```python
from build123d import *

# Parameters (mm, degrees)
SKETCH3_W                       = 80
SKETCH3_H                       = 80
SKETCH3_W_2                     = 60
SKETCH3_H_2                     = 60
BOSS_EXTRUDE2_DEPTH             = 1550
SKETCH7_W                       = 60
SKETCH7_H                       = 60
BOSS_EXTRUDE3_DEPTH             = 5
BOSS_EXTRUDE4_REACH             = 1560.629
SKETCH8_W                       = 110
SKETCH8_H                       = 5
BOSS_EXTRUDE4_DIRECTION_2_REACH = 1560.629
CUT_EXTRUDE1_DEPTH              = 5
CUT_EXTRUDE2_REACH              = 1562.929
FILLET1_R                       = 5
FILLET1_OF_MIRROR1_R            = 5
FILLET1_OF_MIRROR2_R            = 5


with BuildPart() as part:
    # Sketch3 → Boss-Extrude2 (new body)
    with BuildSketch(Plane(origin=(0, 0, 0), x_dir=(0, 0, -1), z_dir=(1, 0, 0))):
        with Locations((40, 40)):
            Rectangle(SKETCH3_W, SKETCH3_H)
        with Locations((40, 40)):
            Rectangle(SKETCH3_W_2, SKETCH3_H_2, mode=Mode.SUBTRACT)
    extrude(amount=BOSS_EXTRUDE2_DEPTH)

    # Sketch7 → Boss-Extrude3 (add)
    with BuildSketch(Plane(origin=(1450, 0, 0), x_dir=(0, 0, -1), z_dir=(1, 0, 0))):
        Polygon((-60, 85), (140, 85), (140, 5), (90, -35), (-10, -35), (-60, 5), align=None)
        with Locations((40, 40)):
            Rectangle(SKETCH7_W, SKETCH7_H, mode=Mode.SUBTRACT)
    boss_extrude3 = extrude(amount=BOSS_EXTRUDE3_DEPTH)

    # Boss-Extrude4: up to this face of the body (flat: up to its plane)
    boss_extrude4_end = Plane(part.part.faces().sort_by_distance((1452.5, 45, -140))[0])
    # Sketch8 → Boss-Extrude4 (add, up to the picked face)
    with BuildSketch(Plane(origin=(0, 0, -80), x_dir=(-1, 0, 0), z_dir=(0, 0, -1)), mode=Mode.PRIVATE) as boss_extrude4_sk1:
        with Locations((-1400, 82.5)):
            Rectangle(SKETCH8_W, SKETCH8_H)
    boss_extrude4_tool1 = split(extrude(boss_extrude4_sk1.sketch, amount=BOSS_EXTRUDE4_REACH, mode=Mode.PRIVATE), bisect_by=boss_extrude4_end, keep=Keep.BOTH, mode=Mode.PRIVATE)
    boss_extrude4 = boss_extrude4_tool1.solids().sort_by(Axis((1400, 82.5, -80), (0, 0, -1)))[0]
    add(boss_extrude4)

    # Boss-Extrude4 direction 2: up to this face of the body (flat: up to its plane)
    boss_extrude4_direction_2_end = Plane(part.part.faces().sort_by_distance((1452.5, 45, 60))[0])
    # Sketch8 → Boss-Extrude4 direction 2 (add, up to the picked face)
    with BuildSketch(Plane(origin=(0, 0, -80), x_dir=(-1, 0, 0), z_dir=(0, 0, -1)), mode=Mode.PRIVATE) as boss_extrude4_direction_2_sk1:
        with Locations((-1400, 82.5)):
            Rectangle(SKETCH8_W, SKETCH8_H)
    boss_extrude4_direction_2_tool1 = split(extrude(boss_extrude4_direction_2_sk1.sketch, amount=-BOSS_EXTRUDE4_DIRECTION_2_REACH, mode=Mode.PRIVATE), bisect_by=boss_extrude4_direction_2_end, keep=Keep.BOTH, mode=Mode.PRIVATE)
    boss_extrude4_direction_2 = boss_extrude4_direction_2_tool1.solids().sort_by(Axis((1400, 82.5, -80), (0, 0, 1)))[0]
    add(boss_extrude4_direction_2)

    # Sketch9 → Cut-Extrude1 (cut)
    with BuildSketch(Plane(origin=(0, 85, 0), x_dir=(1, 0, 0), z_dir=(0, 1, 0))):
        with BuildLine():
            Line((1345, 80), (1350.801257358, 71.298113962))
            ThreePointArc((1350.801257358, 71.298113962), (1353.927300662, 64.675212774), (1355, 57.430609057))
            Line((1355, 57.430609057), (1355, 22.569390943))
            ThreePointArc((1355, 22.569390943), (1353.927300662, 15.324787226), (1350.801257358, 8.701886038))
            Line((1350.801257358, 8.701886038), (1345, 0))
            Line((1345, 0), (1345, 80))
        make_face()
    cut_extrude1 = extrude(amount=-CUT_EXTRUDE1_DEPTH, mode=Mode.SUBTRACT)

    # Sketch10 → Cut-Extrude2 (cut, up to next)
    with BuildSketch(Plane(origin=(0, 85, 0), x_dir=(1, 0, 0), z_dir=(0, 1, 0)), mode=Mode.PRIVATE) as cut_extrude2_sk1:
        with BuildLine():
            Line((1375, 126.5), (1425, 126.5))
            ThreePointArc((1425, 126.5), (1431.5, 120), (1425, 113.5))
            Line((1425, 113.5), (1375, 113.5))
            ThreePointArc((1375, 113.5), (1368.5, 120), (1375, 126.5))
        make_face()
    cut_extrude2_tool1 = extrude(cut_extrude2_sk1.sketch, amount=-CUT_EXTRUDE2_REACH, mode=Mode.PRIVATE) & part.part
    # Sketch10 → Cut-Extrude2 (cut, up to next)
    with BuildSketch(Plane(origin=(0, 85, 0), x_dir=(1, 0, 0), z_dir=(0, 1, 0)), mode=Mode.PRIVATE) as cut_extrude2_sk2:
        with BuildLine():
            Line((1375, -33.5), (1425, -33.5))
            ThreePointArc((1425, -33.5), (1431.5, -40), (1425, -46.5))
            Line((1425, -46.5), (1375, -46.5))
            ThreePointArc((1375, -46.5), (1368.5, -40), (1375, -33.5))
        make_face()
    cut_extrude2_tool2 = extrude(cut_extrude2_sk2.sketch, amount=-CUT_EXTRUDE2_REACH, mode=Mode.PRIVATE) & part.part
    cut_extrude2_1 = cut_extrude2_tool1.solids().sort_by_distance((1400, 85, -120))[0]
    add(cut_extrude2_1, mode=Mode.SUBTRACT)
    cut_extrude2_2 = cut_extrude2_tool2.solids().sort_by_distance((1400, 85, 40))[0]
    add(cut_extrude2_2, mode=Mode.SUBTRACT)
    cut_extrude2 = cut_extrude2_1 + cut_extrude2_2  # Cut-Extrude2 as one shape, for the pattern or mirror that repeats it

    # Fillet1
    fillet1_edges = [part.edges().sort_by_distance(p)[0] for p in [
        (1455, 85, -40),
    ]]
    fillet(fillet1_edges, radius=FILLET1_R - 0.0001)  # a hair under: the kernel refuses the full size

    # Mirror1: Boss-Extrude3 across plane
    add(boss_extrude3.mirror(Plane(origin=(775, 0, 0), x_dir=(0, 0, 1), z_dir=(1, 0, 0))))

    # Fillet1 of Mirror1
    fillet1_of_mirror1_edges = [part.edges().sort_by_distance(p)[0] for p in [
        (95, 85, -40),
    ]]
    fillet(fillet1_of_mirror1_edges, radius=FILLET1_OF_MIRROR1_R - 0.0001)  # a hair under: the kernel refuses the full size

    # Mirror2: Boss-Extrude3, Boss-Extrude4, Boss-Extrude4 direction 2, Cut-Extrude1, Cut-Extrude2 across plane
    add(boss_extrude3.mirror(Plane(origin=(775, 0, 0), x_dir=(0, 0, 1), z_dir=(1, 0, 0))))
    add(boss_extrude4.mirror(Plane(origin=(775, 0, 0), x_dir=(0, 0, 1), z_dir=(1, 0, 0))))
    add(boss_extrude4_direction_2.mirror(Plane(origin=(775, 0, 0), x_dir=(0, 0, 1), z_dir=(1, 0, 0))))
    add(cut_extrude1.mirror(Plane(origin=(775, 0, 0), x_dir=(0, 0, 1), z_dir=(1, 0, 0))), mode=Mode.SUBTRACT)
    add(cut_extrude2.mirror(Plane(origin=(775, 0, 0), x_dir=(0, 0, 1), z_dir=(1, 0, 0))), mode=Mode.SUBTRACT)

    # Fillet1 of Mirror2
    fillet1_of_mirror2_edges = [part.edges().sort_by_distance(p)[0] for p in [
        (95, 85, -40),
    ]]
    fillet(fillet1_of_mirror2_edges, radius=FILLET1_OF_MIRROR2_R - 0.0001)  # a hair under: the kernel refuses the full size


solid = part.part
```
Geometry: final body of the model. Coordinates: model frame, mm. A direction names the side the tool comes from. Give positions to 0.01 mm unless a question says otherwise; leave off trailing zeros. Loops run counter-clockwise (first coordinate to the right, second up) from the corner with the lowest first, then second, coordinate; pieces in that order, holes last. Notation, with made-up numbers: (25.5, 64) -> (40.5, 64) arc R26 cw to (40.5, 89) -> close; hole circle Ø5 at (42, -31). An arc over 180 degrees is marked (long way). Use CSV: the item, a comma, the result in double quotes.
(1) Cut plane B-B (x = 610.5). Output: boundary loops of the cut face in (y, z), plus the area to 3 significant figures.
From the geometry:
outline,"(0, -80) -> (80, -80) -> (80, 0) -> (0, 0) -> close; hole (10, -70) -> (70, -70) -> (70, -10) -> (10, -10) -> close"
area,"2,800 mm^2"
(2) Access query for faces 4 (the face through (1502, 0, -39)), 5 (the face through (764, 40, -70)), 6 (the face through (47, 39, 0)), 7 (the face through (48, 80, -41)). Directions: +Z, -Z, +X, -X, +Y, -Y. A direction counts if a zero-diameter tool reaches every point of the face in a straight line with its end or side. Return the directions, or none.
From the geometry:
face 4,"+Z, -Z, +X, -Y"
face 5,"+X, -X"
face 6,"+Z, -X, +Y, -Y"
face 7,"+Z, -Z, -X, +Y"
(3) Cut plane A-A (y = 44). Output: boundary loops of the cut face in (x, z).
From the geometry:
outline,"(0, -80) -> (95, -80) -> (95, -140) -> (100, -140) -> (100, -80) -> (1450, -80) -> (1450, -140) -> (1455, -140) -> (1455, -80) -> (1550, -80) -> (1550, -70) -> (0, -70) -> close; (0, -10) -> (1550, -10) -> (1550, 0) -> (1455, 0) -> (1455, 60) -> (1450, 60) -> (1450, 0) -> (100, 0) -> (100, 60) -> (95, 60) -> (95, 0) -> (0, 0) -> close"
(4) Pull-direction query (X, two-part tool) for faces 1 (the face through (1502, 39, 0)), 2 (the face through (0, 41, -4)), 3 (the face through (100, -2, -41)); classes: released by +X, released by -X, zero draft, split by the parting line, or undercut.
From the geometry:
face 1,"zero draft"
face 2,"released by -X"
face 3,"undercut"
(5) Ray query, line 1 along Z through (x, y) = (452, 62.5); line 2 along Y through (x, z) = (1181.5, -50); line 3 along X through (y, z) = (-17.5, -46). Return the intervals inside material, ascending. Write a range as [from, to].
From the geometry:
line 1,"[-80, -70], [-10, 0]"
line 2,"[0, 10], [70, 80]"
line 3,"[95, 100], [1450, 1455]"
(6) First-contact query: P1, Ø3, axis at x = 617, y = 58, coming from the -Z side; P2, Ø5.5, axis at y = 83, z = 41, coming from the -X side; P3, Ø18, axis at x = 132.5, z = 39, coming from the -Y side. Flat tips, straight axial feed; report the tip coordinate or a pass-through.
From the geometry:
P1,"z = -80"
P2,"x = 95.01"
P3,"y = 80"
(7) Cut plane C-C (y = -15). Output: boundary loops of the cut face in (x, z).
From the geometry:
outline,"(95, -115) -> (100, -115) -> (100, 35) -> (95, 35) -> close; (1450, -115) -> (1455, -115) -> (1455, 35) -> (1450, 35) -> close"
